The model under review builds one solid part; all positions refer to its coordinate system, in mm. Give positions to 0.01 mm unless a question says otherwise; leave off trailing zeros. Loops run counter-clockwise (first coordinate to the right, second up) from the corner with the lowest first, then second, coordinate; pieces in that order, holes last. Notation, with made-up numbers: M -27.75,77 L 22.25,77 A14 ccw 22.25,83 Z; hole C 43.25,-13 d1. An arc over 180 degrees is marked long. Write item = value, one per line. Start each with the question number.
1. Wall thickness on line 1 along Y through (x, z) = (-27, 3.75); line 2 along X through (y, z) = (-6.5, 6.75); line 3 along X through (y, z) = (1, 7.5): over which ranges is each line inside the solid? List them lowest first. Write a range as from..to.
2. For pin 1 (3 mm diameter, centred on y = 40.5, z = 8, fed in from -X), flat-tipped, find the tip position at first contact; note if it passes through.
3. We need section A-A on y = 18.5. Give the boundary of the cut face in (x, z), then the cut area to 3 significant figures.
4. Draft analysis for pull direction X (two halves, no side actions). For faces 1 (the face through (32.094, -64.719, 3.071)), 2 (the face through (0, -67, 3)), 3 (the face through (-30.45, -62.87, 7.67)), state which applies: pulls with the +X half, pulls with the -X half, needs draft (parallel to the pull), parting line crosses it, or undercut.
from build123d import *

# Parameters (mm, degrees)
F1_DEPTH = 9.2
F2_SIZE  = 4
F3_R     = 1


with BuildPart() as f1:
    # F0 (on Top) → F1 (new body)
    with BuildSketch(Plane.XY):
        with BuildLine():
            Line((26.5, 67), (-26.5, 67))
            ThreePointArc((-26.5, 67), (-32.156854, 64.656854), (-34.5, 59))
            Line((-34.5, 59), (-34.5, -59))
            ThreePointArc((-34.5, -59), (-32.156854, -64.656854), (-26.5, -67))
            Line((-26.5, -67), (26.5, -67))
            ThreePointArc((26.5, -67), (32.156854, -64.656854), (34.5, -59))
            Line((34.5, -59), (34.5, 59))
            ThreePointArc((34.5, 59), (32.156854, 64.656854), (26.5, 67))
        make_face()
    extrude(amount=F1_DEPTH)

    # F2
    f2_edges = [f1.edges().sort_by_distance(p)[0] for p in [
        (-34.5, 0, 9.2),
    ]]
    chamfer(f2_edges, length=F2_SIZE)

    # F3
    f3_edges = [f1.edges().sort_by_distance(p)[0] for p in [
        (34.5, 0, 0),
    ]]
    fillet(f3_edges, radius=F3_R)


solid = f1.part
Final values:
q1.line_1 = -66.98..66.98
q1.line_2 = -32.95..32.95
q1.line_3 = -32.2..32.2
q2.pin_1 = -33.2
q3.outline = M -34.5,1 A1 ccw -33.5,0 L 33.5,0 A1 ccw 34.5,1 L 34.5,5.2 L 30.5,9.2 L -30.5,9.2 L -34.5,5.2 Z
q3.area = 618 mm²
q4.face_1 = pulls with the +X half
q4.face_2 = needs draft
q4.face_3 = pulls with the -X half
